Design review of the part built by this model. Coordinates are the model's own, in mm. Face numbers are marked on the shaded views. A direction names the side the tool comes from. Round coordinates to 2 decimals unless told otherwise and drop trailing zeros. Order: outer loops, then holes, each group sorted by start corner. A loop starts at its lowest first (then second) coordinate and runs counter-clockwise, first axis right, second up. Notation, with made-up numbers: M 77,-35.5 L 127,-35.5 A23 cw 127,-18.5 Z; hole C -36,79.5 d4. An arc over 180 degrees is marked long. Write item = value, one per line. Start each with the question number.
Autodesk Inventor part; units mm, degrees
ref_plane "Work Plane1" through (20, 0, 0) normal (0, 0.5, 0.866) x (1, 0, 0)
ref_plane "YZ Plane" through (0, 0, 0) normal (1, 0, 0) x (0, 1, 0)
ref_plane "XZ Plane" through (0, 0, 0) normal (0, 1, 0) x (-1, 0, 0)
sketch "Esquisse1" plane through (0, 0, 0) normal (0, 0, 1) x (1, 0, 0)
  line L0 (1.2217, 0) -> (40, 0)
  line L1 (40, 0) -> (40, 2.5)
  line L2 (40, 2.5) -> (0, 2.5)
  line L3 (0, 2.5) -> (0, 4.25)
  line L4 (0, 4.25) -> (-3.5, 4.25)
  line L5 (-3.5, 4.25) -> (-3.5, 2.3094)
  line L6 (-3.5, 2.3094) -> (-1.5, 2.3094)
  line L7 (-1.5, 2.3094) -> (-0.8884, 1.25)
  line L8 (-12.2, 0) -> (48.7, 0)
  line L9 (0, -0.85) -> (0, 5.1)
  line L10 (-0.8884, 1.25) -> (0.5, 1.25)
  line L11 (0.5, 1.25) -> (1.2217, 0)
  line L12 (-3.5, 2.3094) -> (-3.5, 0) construction
  line L13 (-3.5, 3.75) -> (-3, 4.25)
  dimension "d0" = 3.5
  dimension "d1" = 2
  dimension "d2" = 60
  dimension "d3" = 5
  dimension "d4" = 4.6188
  dimension "d5" = 8.5
  dimension "d15" = 4
  dimension "d16" = 2.5
  dimension "d17" = 40
  dimension "d32" = 45
  dimension "d33" = 0.5
revolve "Corps" add sketch "Esquisse1" angle 360 about axis through (1.2217, 0, 0) along (1, 0, 0) contours L11 L10 L9 L2 L1 L0 | L10 L7 L6 L5 L13 L4 L3 L9 | L13 L5 L4
revolve "Chanfrein2" cut sketch "Esquisse1" angle 360 about axis through (-10, 0, 0) along (1, 0, 0) contours L13 L5 L4
sketch "Esquisse2" plane through (-3.5, 0, 0) normal (-1, 0, 0) x (0, 0, 1)
  circle A0 centre (0, 0) radius 2.3094
  line L0 (0, -5.95) -> (0, 5.95)
  line L1 (-5.95, 0) -> (5.95, 0)
  line L2 (2.3094, 0) -> (1.1547, -2)
  line L3 (1.1547, -2) -> (-1.1547, -2)
  line L4 (-1.1547, -2) -> (-2.3094, 0)
  line L5 (-2.3094, 0) -> (-1.1547, 2)
  line L6 (-1.1547, 2) -> (1.1547, 2)
  line L7 (1.1547, 2) -> (2.3094, 0)
extrude "Rainure" add sketch "Esquisse2" against normal up to next contours L7 A0 | A0 L2 | L6 L0 A0 | A0 L0 L3 | L0 L6 A0 | A0 L3 L0 | L4 A0 | A0 L5
thread "Filetage"
chamfer "Chanfrein1" distance 0.4908 distance2 0.4908 1 edges at (40, -2.5, 0) measured on face at (40, 0.9945, 0.5526)
ref_plane "Work Plane1" through (20, 0, 0) normal (0, 0.5, 0.866) x (1, 0, 0)
equation "\"d0\" = KOH"
equation "\"d1\" = INTI"
equation "\"d3\" = GD"
equation "\"d4\" = 1.1547 * SW"
equation "\"d5\" = KOD"
equation "\"d15\" = INFT"
equation "\"d16\" = SDT"
equation "\"d17\" = NLG"
equation "\"d33\" = Cham"
equation "\"d7\" = GEL"
equation "\"d9\" = -0.5 * SPD + 0.5 * GD"
equation "\"d12\" = GUL"
equation "\"GD\" = NND"
equation "\"NLG\" = 40"
equation "\"GEL\" = 16"
equation "\"KOD\" = 8.5"
equation "\"KOH\" = 3.5"
equation "\"GUL\" = 0.61345 * PTC"
equation "\"SW\" = 4"
equation "\"INTI\" = 2"
equation "\"SPD\" = NND - 1.2269 * PTC"
equation "\"SDT\" = 2.5"
equation "\"INFT\" = 4"
equation "\"Cham\" = 0.5"
equation "\"TOA\" = 30deg"
equation "\"GD1\" = THREADDIA - 1.2269 * PTC"
equation "\"THREADDIA\" = 5"
equation "\"BDM\" = NND"
equation "\"FAWI\" = 45deg"
equation "\"RR\" = 0.1 * NND"
equation "\"PTC\" = 0.8"
equation "\"NND\" = 5"
equation "\"FAWI1\" = 45deg"
equation "\"GAL\" = 0.61345 * PTC"
equation "\"E0\" = 1.155 * SW"
properties part number "DIN 6912 - M5 x 40" material "Acier, doux"
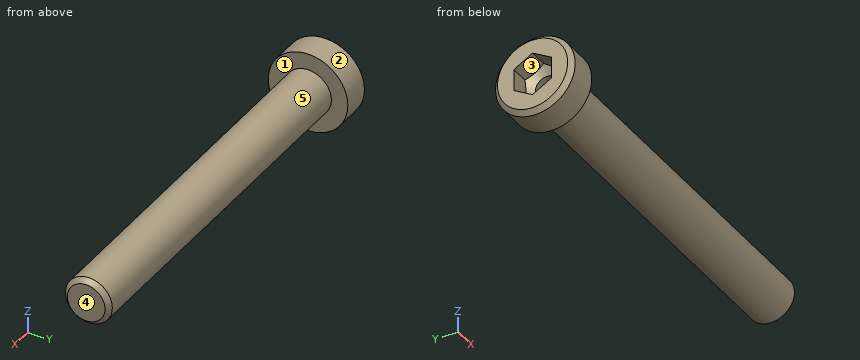
(1) Consider section A-A, the plane x = 16. Write out the cut boundary in (y, z), then the cut area to 3 significant figures.
(2) For line 1 along Z through (x, y) = (0.15, 0); line 2 along Z through (x, y) = (-0.2, 0); line 3 along X through (y, z) = (2.75, 1.75), list the stretches that pass through material, from the lowest coordinate up. Write a range as [from, to].
(3) For the marked faces 1 and 2, list the 3-axis set-ups (+Z, -Z, +X, -X, +Y, -Y) from which the entire face can be reached by the end or side of a thin tool; tool diameter is ignored.
(4) Draft analysis for pull direction Z (two halves, no side actions). For the marked faces 3, 4 and 5, state which applies: pulls with the +Z half, pulls with the -Z half, needs draft (parallel to the pull), parting line crosses it, or undercut.
(5) Insertion check: pin 1 (5 mm diameter, centred on x = 19.5, z = -1.5, fed in from +Y); pin 2 (2 mm diameter, centred on x = 26, y = 2, fed in from +Z). Each pin has a flat end and moves straight along its axis. Give the tip position at first contact, or say it passes through.
Completed:
q1.outline = C 0,0 d5
q1.area = 19.6 mm2
q2.line_1 = [-2.5, -1.25], [1.25, 2.5]
q2.line_2 = [-4.25, -1.25], [1.25, 4.25]
q2.line_3 = [-3.5, 0]
q3.face_1 = +X
q3.face_2 = +X, -X
q4.face_3 = undercut
q4.face_4 = needs draft
q4.face_5 = parting line crosses it
q5.pin_1 = 2.5
q5.pin_2 = 2.29
